```python
from build123d import *

# Parameters (mm, degrees)
BOSS_EXTRUDE1_DEPTH  = 5.5
CHASSIS_WALLS1_DEPTH = 8
CHAMFER1_SIZE        = 10
CHAMFER2_SIZE        = 10
CHAMFER3_SIZE        = 2.5
SKETCH4_R            = 2.4
CUT_EXTRUDE1_DEPTH   = 10
SKETCH5_W            = 55
SKETCH5_H            = 8
CUT_EXTRUDE2_DEPTH   = 10
SKETCH6_W            = 65
SKETCH6_H            = 5
CUT_EXTRUDE3_DEPTH   = 6.5


with BuildPart() as part:
    # Sketch1 → Boss-Extrude1 (new body)
    with BuildSketch(Plane(origin=(0, 0, 0), x_dir=(1, 0, 0), z_dir=(0, 1, 0))):
        Polygon((-100, 36.25), (-70, 55), (70, 55), (100, 32.5), (175, 32.5), (175, -32.5), (100, -32.5), (70, -55), (-70, -55), (-100, -36.25), (-160, -36.25), (-160, 36.25), align=None)
    extrude(amount=BOSS_EXTRUDE1_DEPTH)

    # Sketch3 → Chassis-Walls1 (add)
    with BuildSketch(Plane(origin=(0, 5.5, 0), x_dir=(1, 0, 0), z_dir=(0, 1, 0))):
        Polygon((0, 55), (-70, 55), (-100, 36.25), (-97.88000424, 32.858006784), (-67.88000424, 51.608006784), (0, 51.608006784), (67.456005088, 51.608006784), (97.456005088, 29.108006784), (100, 32.5), (70, 55), align=None)
        Polygon((67.456005088, -51.608006784), (0, -51.608006784), (-67.88000424, -51.608006784), (-97.88000424, -32.858006784), (-100, -36.25), (-70, -55), (0, -55), (70, -55), (100, -32.5), (97.456005088, -29.108006784), align=None)
    extrude(amount=CHASSIS_WALLS1_DEPTH)

    # Chamfer1
    chamfer1_edges = [part.edges().sort_by_distance(p)[0] for p in [
        (-160, 2.75, 36.25),
        (-160, 2.75, -36.25),
    ]]
    chamfer(chamfer1_edges, length=CHAMFER1_SIZE)

    # Chamfer2
    chamfer2_edges = [part.edges().sort_by_distance(p)[0] for p in [
        (175, 2.75, -32.5),
        (175, 2.75, 32.5),
    ]]
    chamfer(chamfer2_edges, length=CHAMFER2_SIZE)

    # Chamfer3
    chamfer3_edges = [part.edges().sort_by_distance(p)[0] for p in [
        (-98.94000212, 13.5, -34.554003392),
        (98.728002544, 13.5, -30.804003392),
        (-98.94000212, 13.5, 34.554003392),
        (98.728002544, 13.5, 30.804003392),
    ]]
    chamfer(chamfer3_edges, length=CHAMFER3_SIZE)

    # Sketch4 → Cut-Extrude1 (cut)
    with BuildSketch(Plane.XZ):
        with Locations((-152, 17)):
            Circle(SKETCH4_R)
        with Locations((-60, 17)):
            Circle(SKETCH4_R)
        with Locations((-60, -17)):
            Circle(SKETCH4_R)
        with Locations((-152, -17)):
            Circle(SKETCH4_R)
        with Locations((-30, 31)):
            Circle(SKETCH4_R)
        with Locations((55, 31)):
            Circle(SKETCH4_R)
        with Locations((55, -31)):
            Circle(SKETCH4_R)
        with Locations((-30, -31)):
            Circle(SKETCH4_R)
    extrude(amount=-CUT_EXTRUDE1_DEPTH, mode=Mode.SUBTRACT)

    # Sketch5 → Cut-Extrude2 (cut)
    with BuildSketch(Plane(origin=(0, 5.5, 0), x_dir=(1, 0, 0), z_dir=(0, 1, 0))):
        with Locations((-132.5, -32.25)):
            Rectangle(SKETCH5_W, SKETCH5_H)
    extrude(amount=-CUT_EXTRUDE2_DEPTH, mode=Mode.SUBTRACT)

    # Sketch6 → Cut-Extrude3 (cut, through all)
    with BuildSketch(Plane(origin=(0, 5.5, 0), x_dir=(1, 0, 0), z_dir=(0, 1, 0))):
        with Locations((12.5, 22.5)):
            Rectangle(SKETCH6_W, SKETCH6_H)
        with Locations((12.5, -22.5)):
            Rectangle(SKETCH6_W, SKETCH6_H)
    extrude(amount=-CUT_EXTRUDE3_DEPTH, mode=Mode.SUBTRACT)


solid = part.part
```
Model file for the job. Use its own axes, mm. A direction names the side the tool comes from. Give positions to 0.01 mm unless a question says otherwise; leave off trailing zeros. Order: outer loops, then holes, each group sorted by start corner. A loop starts at its lowest first (then second) coordinate and runs counter-clockwise, first axis right, second up.
1) Pin check, flat tips, straight feed: pin 1 (6 mm diameter, centred on x = 126, y = 1.5, fed in from +Z); pin 2 (5 mm diameter, centred on x = 73, y = 5, fed in from +Z) (3 decimals); pin 3 (1.6 mm diameter, centred on x = -119, y = 1.5, fed in from -Z); pin 4 (3 mm diameter, centred on x = 55, z = 31, fed in from +Y). Stop position of each tip, or through.
2) Saw through at B-B, the plane z = -1.5. Write the cut outline in (x, y), then the cut area to 3 significant figures.
3) Wall check: probe 1 along Z at (x, y) = (-60, 3.45); probe 2 along Z at (x, y) = (8, 4); probe 3 along Z at (x, y) = (53.5, 11.5). Give the ranges that are in metal, low to high.
4) Saw through at C-C, the plane x = 84. Write the cut outline in (y, z), then the cut area to 3 significant figures.
5) 3-axis set-ups, long thin cutter, end or side, ignore diameter. For faces 1 (the flat face through (1, 7, -55)), 2 (the flat face through (-125, 3, -36.25)), 3 (the flat face through (170.1, 2.7, 27.4)), 4 (the flat face through (10, 5.5, -1)), 5 (the flat face through (12, 3, -20)): which of +Z, -Z, +X, -X, +Y, -Y reach the whole face in a straight line?
6) Saw through at A-A, the plane x = 13. Write the cut outline in (y, z).
7) Mould opens along X. For faces 6 (the flat face through (-105, 3, 32)), 7 (the flat face through (-82.67, 9.444, 42.364)), 8 (the flat face through (85.2, 6.7, 43.6)), 9 (the flat face through (-83.09, 9.44, -42.1)) say: +X half, -X half, draft (parallel to the pull), parting line (faces both ways), or undercut.
8) Saw through at D-D, the plane x = -124. Write the cut outline in (y, z).
Computed:
1. pin 1: stops at z = 32.5
1. pin 2: stops at z = 54.625
1. pin 3: stops at z = -36.25
1. pin 4: passes through
2. outline: (-160, 0) - (175, 0) - (175, 5.5) - (-160, 5.5) - close
2. area: 1,840 mm2
3. probe 1: z = -55 to -19.4, -14.6 to 14.6, 19.4 to 55
3. probe 2: z = -55 to -25, -20 to 20, 25 to 55
3. probe 3: z = -55 to -51.61, 51.61 to 55
4. outline: (0, -44.5) - (13.5, -44.5) - (13.5, -39.2) - (5.5, -39.2) - (5.5, 39.2) - (13.5, 39.2) - (13.5, 44.5) - (0, 44.5) - close
4. area: 574 mm2
5. face 1: -Z, +X, -X, +Y, -Y
5. face 2: -Z, -X, +Y, -Y
5. face 3: +Z, +X, +Y, -Y
5. face 4: +Y
5. face 5: +Y, -Y
6. outline: (0, -55) - (13.5, -55) - (13.5, -51.61) - (5.5, -51.61) - (5.5, -25) - (0, -25) - close; (0, -20) - (5.5, -20) - (5.5, 20) - (0, 20) - close; (0, 25) - (5.5, 25) - (5.5, 51.61) - (13.5, 51.61) - (13.5, 55) - (0, 55) - close
7. face 6: -X half
7. face 7: undercut
7. face 8: +X half
7. face 9: undercut
8. outline: (0, -36.25) - (5.5, -36.25) - (5.5, 28.25) - (0, 28.25) - close
